Geometry: see drawing. Coordinates: mm, zero at the bounding-box minimum. A direction names the side the tool comes from. Coordinates: 2 decimals unless noted, no trailing zeros. Order: outer loops, then holes, each group sorted by start corner. A loop starts at its lowest first (then second) coordinate and runs counter-clockwise, first axis right, second up. Notation, with made-up numbers: (12, -17) -> (24, -17) arc R4 cw to (24, -11) -> close; hole circle Ø5 at (36, 25.25). An arc over 180 degrees is marked (long way). Write each question's results on one line, items separated by ' | '.
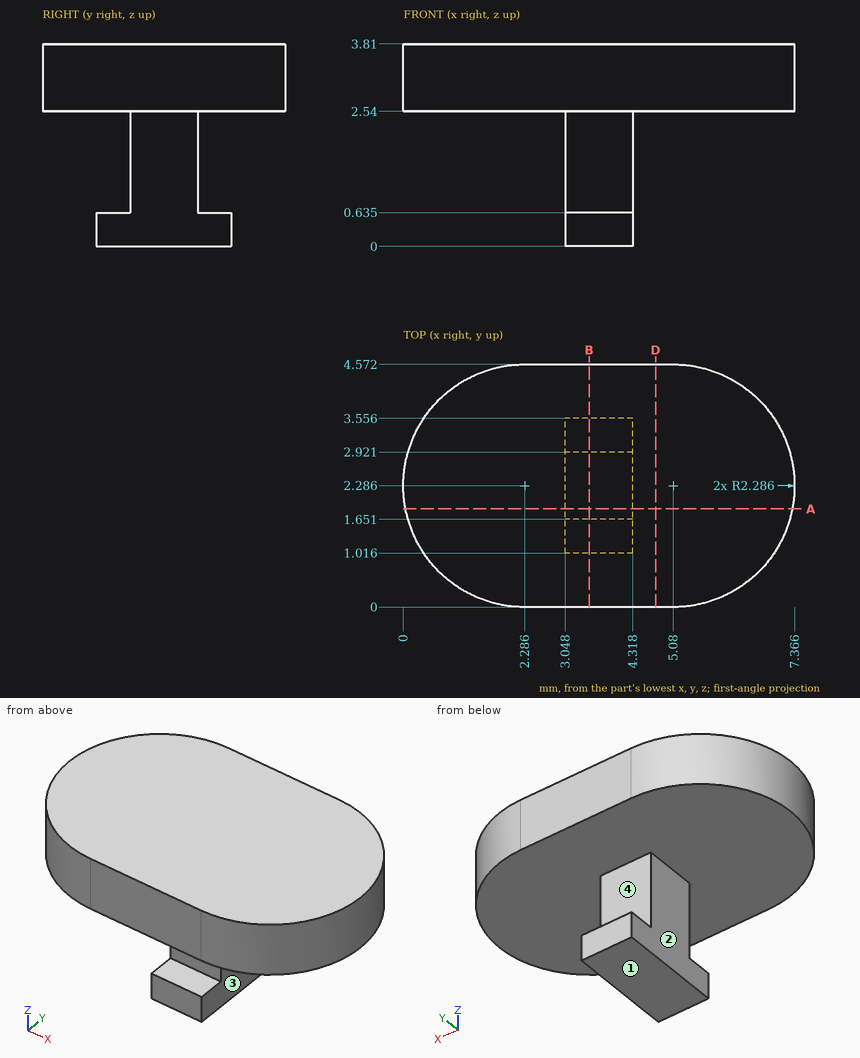
(1) Reachability of the marked faces 1, 2, 3 and 4 from +Z, -Z, +X, -X, +Y, -Y: full face, straight path, thin tool, end or side. Return the list, or none.
Return value:
face 1: -Z, +X, -X, +Y, -Y | face 2: -Z, -X, +Y, -Y | face 3: -Z, +X, +Y, -Y | face 4: +X, -X, +Y
(2) Pin query (flat end, axial travel): P1, Ø2, axis at y = 0.5, z = 2.5, coming from the +X side; P2, Ø1, axis at x = 4, z = 1, coming from the +Y side; P3, Ø2, axis at x = 1, z = 2.5, coming from the -Y side. Return the tip coordinate at first contact, or that it passes through.
Return value:
P1: x = 7.23 | P2: y = 3.56 | P3: y = 0.02
(3) Cut plane B-B, the plane x = 3.5. Return loops of the section in (y, z) (3 decimals).
Return value:
outline: (0, 2.54) -> (1.651, 2.54) -> (1.651, 0.635) -> (1.016, 0.635) -> (1.016, 0) -> (3.556, 0) -> (3.556, 0.635) -> (2.921, 0.635) -> (2.921, 2.54) -> (4.572, 2.54) -> (4.572, 3.81) -> (0, 3.81) -> close
(4) Cut plane D-D, the plane x = 4.75. Return loops of the section in (y, z).
Return value:
outline: (0, 2.54) -> (4.57, 2.54) -> (4.57, 3.81) -> (0, 3.81) -> close
(5) Line query: line 1 along Z through (x, y) = (2, 1.6); line 2 along X through (y, z) = (3.3, 0.4); line 3 along X through (y, z) = (3, 2.6). Output: solid intervals per line, ascending. Write a range as from..to.
Return value:
line 1: 2.54..3.81 | line 2: 3.05..4.32 | line 3: 0.11..7.25
(6) Cut plane A-A, the plane y = 1.85. Return loops of the section in (x, z), plus the area to 3 significant figures.
Return value:
outline: (0.04, 2.54) -> (3.05, 2.54) -> (3.05, 0) -> (4.32, 0) -> (4.32, 2.54) -> (7.32, 2.54) -> (7.32, 3.81) -> (0.04, 3.81) -> close | area: 12.5 mm2
